from build123d import *

# Parameters (mm, degrees)
F0_R        = 10
F1_DEPTH    = 25
F2_DEPTH    = 50
F3_T4_ANGLE = 203.6133668192
F3_T8_ANGLE = 190.697258089


# Not quite as in the source:
# - a fillet or chamfer that OpenCascade refuses, or shapes differently, is made with other operations: its cross-section is extruded or revolved along the edge and cut away or added


with BuildPart() as f1:
    # F0 (on Front) → F1 (new body)
    with BuildSketch(Plane.XZ):
        with BuildLine():
            Line((2.8107571296, 24.8414903812), (0, 25))
            ThreePointArc((0, 25), (-25, 0), (0, -25))
            Line((0, -25), (2.8107571296, -24.8414903812))
            ThreePointArc((2.8107571296, -24.8414903812), (18.6449581421, -16.6542948179), (25, 0))
            ThreePointArc((25, 0), (18.6449581421, 16.6542948179), (2.8107571296, 24.8414903812))
        make_face()
        Circle(F0_R, mode=Mode.SUBTRACT)
        with BuildLine():
            Line((133.4853280749, 17.4722387972), (2.8107571296, 24.8414903812))
            ThreePointArc((2.8107571296, 24.8414903812), (18.6449581421, 16.6542948179), (25, 0))
            ThreePointArc((25, 0), (18.6449581421, -16.6542948179), (2.8107571296, -24.8414903812))
            Line((2.8107571296, -24.8414903812), (133.4853280749, -17.4722387972))
            ThreePointArc((133.4853280749, -17.4722387972), (115, 0), (133.4853280749, 17.4722387972))
        make_face()
        with BuildLine():
            ThreePointArc((150, 0), (145.2179644855, 12.0209558415), (133.4853280749, 17.4722387972))
            ThreePointArc((133.4853280749, 17.4722387972), (115, 0), (133.4853280749, -17.4722387972))
            ThreePointArc((133.4853280749, -17.4722387972), (145.2179644855, -12.0209558415), (150, 0))
        make_face()
        with Locations((132.5, 0)):
            Circle(F0_R, mode=Mode.SUBTRACT)
    extrude(amount=F1_DEPTH)

    # F0 (on Front) → F2 (join)
    with BuildSketch(Plane.XZ):
        with BuildLine():
            Line((2.8107571296, 24.8414903812), (0, 25))
            ThreePointArc((0, 25), (-25, 0), (0, -25))
            Line((0, -25), (2.8107571296, -24.8414903812))
            ThreePointArc((2.8107571296, -24.8414903812), (18.6449581421, -16.6542948179), (25, 0))
            ThreePointArc((25, 0), (18.6449581421, 16.6542948179), (2.8107571296, 24.8414903812))
        make_face()
        Circle(F0_R, mode=Mode.SUBTRACT)
    extrude(amount=F2_DEPTH)

    # F3: chamfer of 2 on 4 edges, made by hand

    # F3_s1 → F3_t2 (revolve, cut)
    with BuildSketch(Plane.XY):
        Polygon((10, -48), (12, -50), (10, -50), align=None)
    revolve(axis=Axis((0, -50, 0), (0, -1, 0)), mode=Mode.SUBTRACT)

    # F3_s3 → F3_t4 (revolve, cut)
    with BuildSketch(Plane(origin=(0, 0, 0), x_dir=(0, 1, 0), z_dir=(0.9788435281, 0, -0.2046102329))):
        Polygon((-48, 25), (-50, 23), (-50, 25), align=None)
    revolve(axis=Axis((0, -50, 0), (0, -1, 0)), revolution_arc=F3_T4_ANGLE, mode=Mode.SUBTRACT)

    # F3_s5 → F3_t6 (revolve, cut)
    with BuildSketch(Plane.XY):
        Polygon((142.5, -23), (144.5, -25), (142.5, -25), align=None)
    revolve(axis=Axis((132.5, -25, 0), (0, -1, 0)), mode=Mode.SUBTRACT)

    # F3_s7 → F3_t8 (revolve, cut)
    with BuildSketch(Plane(origin=(0, 0, 0), x_dir=(0, 1, 0), z_dir=(-0.9956459412, 0, -0.0932156624))):
        Polygon((-48, -25), (-50, -23), (-50, -25), align=None)
    revolve(axis=Axis((0, -50, 0), (0, 1, 0)), revolution_arc=F3_T8_ANGLE, mode=Mode.SUBTRACT)


solid = f1.part
CAD build for the part. Positions are in the model's coordinates, mm. Coordinates: 2 decimals unless noted, no trailing zeros. Loops run counter-clockwise (first coordinate to the right, second up) from the corner with the lowest first, then second, coordinate; pieces in that order, holes last. Notation, with made-up numbers: (68, -7.75) - (73, -7.75) arc R31 ccw to (73, 27.25) - close; hole circle Ø2 at (45.25, -13). An arc over 180 degrees is marked (long way). Write item = value, one per line. Start each with the question number.
Q1. Pull direction Z, two halves, no side cores. Call faces 1 (the cylindrical face through (-24.994, -23.664, 0.55)), 2 (the conical face through (141.853, -23.125, -3.878)), 3 (the flat face through (61, 0, 0)): pulls with the +Z half, pulls with the -Z half, needs draft (parallel to the pull), parting line crosses it, or undercut.
Q2. Cut at A-A, the plane y = -37. List the corners of the cut face in (x, z), then the cut area to 3 significant figures.
Q3. Flat gauge pins, fed straight in: pin 1 Ø4 at (x, y) = (50, -6) entering from -Z; pin 2 Ø4 at (x, y) = (116.5, -17.5) entering from -Z; pin 3 Ø15 at (x, z) = (98, -11.5) entering from -Y. Where does each tip first touch, or does it go through?
Q4. Drill centre lines: L1, parallel to X at y = -40.5, z = -0.5 (1 decimal); L2, parallel to Y at x = 96, z = -12.5; L3, parallel to Z at x = 132, y = -6. Where is each one in solid material? Low to high.
Q5. Cut at D-D, the plane x = 85.5. List the corners of the cut face in (y, z), then the cut area to 3 significant figures.
Q6. Cut at B-B, the plane y = -20.5. List the corners of the cut face in (x, z).
Q7. Cut at C-C, the plane z = -2. Give the number of separate pieces and of enclosed holes in the cut face, then the cut area to 3 significant figures.
Computed:
q1.face_1 = parting line crosses it
q1.face_2 = undercut
q1.face_3 = needs draft
q2.outline = (0, -25) - (2.81, -24.84) arc R25 ccw to (2.81, 24.84) - (0, 25) arc R25 ccw to start; hole circle Ø20 at (0, 0)
q2.area = 1,650 mm²
q3.pin_1 = -22.29
q3.pin_2 = -18.54
q3.pin_3 = -25
q4.L1 = -25 to -10, 10 to 25
q4.L2 = -25 to 0
q4.L3 = -17.56 to -9.99, 9.99 to 17.56
q5.outline = (-25, -20.18) - (0, -20.18) - (0, 20.18) - (-25, 20.18) - close
q5.area = 1,010 mm²
q6.outline = (0, -25) - (133.49, -17.47) arc R17.5 ccw to (133.49, 17.47) - (0, 25) arc R25 ccw to start; hole circle Ø20 at (0, 0); hole circle Ø20 at (132.5, 0)
q7.separate_pieces = 3
q7.enclosed_holes = 0
q7.area = 4,130 mm²
